Read the model definition and answer for the solid it produces. Units are mm, in the model's axes. Coordinates: 2 decimals unless noted, no trailing zeros. Loops run counter-clockwise (first coordinate to the right, second up) from the corner with the lowest first, then second, coordinate; pieces in that order, holes last. Notation, with made-up numbers: (-11, 12) -> (48, 12) arc R11 ccw to (48, 31) -> close; hole circle Ø11 at (26, 89.5). An arc over 180 degrees is marked (long way). Answer as a JSON object with one key per item and string values. Group by question number.
1) Section B-B, the plane y = 56.5 is taken. Give the vertices of the cut face in (x, z), plus the area to 3 significant figures.
2) Section A-A, the plane y = -3.75 is taken. Give the vertices of the cut face in (x, z), plus the area to 3 significant figures.
3) Section D-D, the plane x = 37.5 is taken. Give the vertices of the cut face in (y, z), plus the area to 3 significant figures.
4) Section C-C, the plane x = 19 is taken. Give the vertices of the cut face in (y, z), plus the area to 3 significant figures.
5) Consider probe 1 along X at (y, z) = (-4, 0.4); probe 2 along Y at (x, z) = (65, 0.2); probe 3 along Y at (x, z) = (21.5, 0.45). Determine where each line is inside the solid, lowest interval first. Write a range as [from, to].
from build123d import *

# Parameters (mm, degrees)
EXTRUDE_DEPTH = 1
SKETCH001_R   = 1.1
HOLE_DEPTH    = 5
SKETCH002_R   = 1.65
HOLE001_DEPTH = 3


with BuildPart() as part:
    # Sketch → Extrude (new body)
    with BuildSketch(Plane.XY):
        Polygon((0, 0), (5, 0), (5, -7.5), (12.5, -7.5), (12.5, 0), (33.75, 0), (33.75, -7.5), (41.25, -7.5), (41.25, 0), (62.5, 0), (62.5, -7.5), (70, -7.5), (70, 0), (75, 0), (75, 7.5), (50, 7.5), (50, 18), (62, 18), (72.500012, 25.352225), (72.500012, 35), (43.500012, 35), (43.500012, 60.5), (31.500012, 60.5), (31.500012, 35), (2.500012, 35), (2.499988, 25.352225), (13, 18), (25, 18), (25, 7.5), (0, 7.5), align=None)
    extrude(amount=EXTRUDE_DEPTH)

    # Sketch001 (on Face32 of Extrude) → Hole (cut)
    with BuildSketch(Plane.XY.offset(1)):
        with Locations((2.5, 5)):
            Circle(SKETCH001_R)
        with Locations((15.3, 5)):
            Circle(SKETCH001_R)
        with Locations((59.7, 5)):
            Circle(SKETCH001_R)
        with Locations((72.5, 5)):
            Circle(SKETCH001_R)
    extrude(amount=-HOLE_DEPTH, mode=Mode.SUBTRACT)

    # Sketch002 (on Face5 of Hole) → Hole001 (cut)
    with BuildSketch(Plane.XY.offset(1)):
        with Locations((8.75, -3.75)):
            Circle(SKETCH002_R)
        with Locations((37.5, -3.75)):
            Circle(SKETCH002_R)
        with Locations((66.25, -3.75)):
            Circle(SKETCH002_R)
        with Locations((37.5, 56.5)):
            Circle(SKETCH002_R)
    extrude(amount=-HOLE001_DEPTH, mode=Mode.SUBTRACT)


solid = part.part
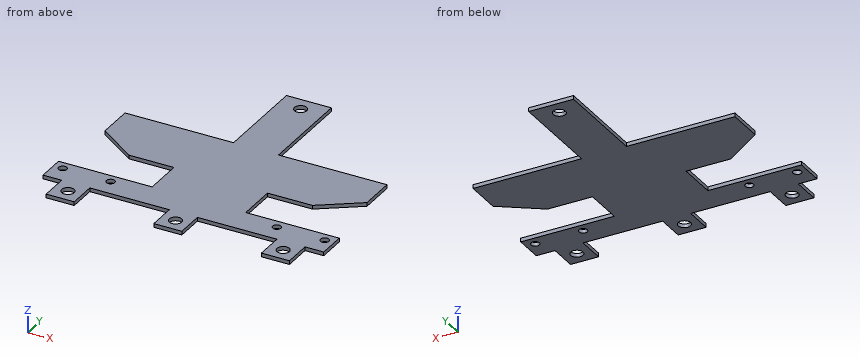
Determined:
{
 "1": {"outline": "(31.5, 0) -> (35.85, 0) -> (35.85, 1) -> (31.5, 1) -> close; (39.15, 0) -> (43.5, 0) -> (43.5, 1) -> (39.15, 1) -> close", "area": "8.70 mm²"},
 "2": {"outline": "(5, 0) -> (7.1, 0) -> (7.1, 1) -> (5, 1) -> close; (10.4, 0) -> (12.5, 0) -> (12.5, 1) -> (10.4, 1) -> close; (33.75, 0) -> (35.85, 0) -> (35.85, 1) -> (33.75, 1) -> close; (39.15, 0) -> (41.25, 0) -> (41.25, 1) -> (39.15, 1) -> close; (62.5, 0) -> (64.6, 0) -> (64.6, 1) -> (62.5, 1) -> close; (67.9, 0) -> (70, 0) -> (70, 1) -> (67.9, 1) -> close", "area": "12.6 mm²"},
 "3": {"outline": "(-7.5, 0) -> (-5.4, 0) -> (-5.4, 1) -> (-7.5, 1) -> close; (-2.1, 0) -> (54.85, 0) -> (54.85, 1) -> (-2.1, 1) -> close; (58.15, 0) -> (60.5, 0) -> (60.5, 1) -> (58.15, 1) -> close", "area": "61.4 mm²"},
 "4": {"outline": "(0, 0) -> (7.5, 0) -> (7.5, 1) -> (0, 1) -> close; (18, 0) -> (35, 0) -> (35, 1) -> (18, 1) -> close", "area": "24.5 mm²"},
 "5": {"probe 1": "[5, 7.12], [10.38, 12.5], [33.75, 35.87], [39.13, 41.25], [62.5, 64.62], [67.88, 70]", "probe 2": "[-7.5, -4.83], [-2.67, 7.5], [20.1, 35]", "probe 3": "[0, 7.5], [18, 35]"}
}
